CAD build for the part. Positions are in the model's coordinates, mm. Coordinates: 2 decimals unless noted, no trailing zeros. Write each loop counter-clockwise with the first axis right and the second up, starting at its lowest first coordinate (ties: lowest second). Pieces come first, ordered by that corner, then holes. Notation, with made-up numbers: (-13, -16.75) - (18, -16.75) arc R27 cw to (18, 6.25) - close; hole circle Ø5 at (29.25, 57). An arc over 180 degrees is marked (long way). Answer in a Markdown table with one row per item. Add a question column.
Q1. Pin check, flat tip, straight feed: pin 1 (1 mm diameter, centred on y = -1, z = 10.5, fed in from +X). Stop position of the tip, or through.
Q2. Band-saw the part on A-A (z = 18.75). List the corners of the cut face in (x, y).
Q3. Band-saw the part on C-C (y = 0.45). List the corners of the cut face in (x, z), and give its area (3 significant figures).
Q4. Band-saw the part on B-B (x = 0.3). List the corners of the cut face in (y, z), and give its area (3 significant figures).
Q5. Drill centre lines: line 1 along Y through (x, z) = (0.05, 20.5); line 2 along Y through (x, z) = (-0.7, 16). Where is each one in solid material? Low to high. Write a range as from..to.
Autodesk Fusion 360 part; units mm, degrees
sketch "Boceto1" plane through (0, 0, 0) normal (0, 0, 1) x (1, 0, 0)
  line L0 (0, 0) -> (120, 0)
  line L1 (120, 0) -> (120, 50)
  line L2 (120, 50) -> (0, 50)
  line L3 (0, 50) -> (0, 0)
  dimension "d1" = 120
  dimension "d2" = 50
extrude "Extruir1" add sketch "Boceto1" along normal blind 3
sketch "Boceto2" plane through (0, 0, 3) normal (0, 0, 1) x (-1, 0, 0)
  line L0 (0, -50) -> (0, 0)
  line L1 (0, 0) -> (-120, 0)
  line L2 (-120, 0) -> (-120, -50)
  line L3 (-120, -50) -> (0, -50)
  line L4 (-120, -25) -> (0, -25)
  line L5 (-120, -25) -> (-100, -25)
  circle A0 centre (-100, -25) radius 3
  line L6 (-100, -25) -> (-83.13, -25)
  circle A1 centre (-83.13, -25) radius 3
  line L7 (-83.13, -25) -> (-66.26, -25)
  circle A2 centre (-66.26, -25) radius 3
  line L8 (-66.26, -25) -> (-49.39, -25)
  circle A3 centre (-49.39, -25) radius 3
  line L9 (-49.39, -25) -> (-32.52, -25)
  circle A4 centre (-32.52, -25) radius 3
  line L10 (-32.52, -25) -> (-15.65, -25)
  circle A5 centre (-15.65, -25) radius 3
  dimension "d5" = 20
  dimension "d6" = 6
  dimension "d7" = 16.87
  dimension "d8" = 6
  dimension "d9" = 16.87
  dimension "d11" = 6
  dimension "d12" = 16.87
  dimension "d13" = 6
  dimension "d14" = 16.87
  dimension "d15" = 6
  dimension "d16" = 16.87
  dimension "d17" = 6
extrude "Extruir2" cut sketch "Boceto2" against normal blind 3 contours L4 L10 A5 | L4 L10 A5 | L4 L5 A0 L6 | L4 L5 A0 L6 | L4 L9 A4 L10 | L4 L9 A4 L10 | L4 L6 A1 L7 | L4 L6 A1 L7 | L4 L8 A3 L9 | L4 L8 A3 L9 | L4 L7 A2 L8 | L4 L7 A2 L8
equation "d6 = D_b"
equation "d7 = Dc"
equation "d8 = D_b"
equation "d9 = Dc"
equation "Dc = 16.87 mm"
equation "d11 = D_b"
equation "d12 = Dc"
equation "d13 = D_b"
equation "d14 = Dc"
equation "d15 = D_b"
equation "d16 = Dc"
equation "d17 = D_b"
equation "D_b = 6 mm"

Autodesk Fusion 360 part; units mm, degrees
sketch "Boceto1" plane through (0, 0, 0) normal (0, 0, 1) x (1, 0, 0)
  circle A0 centre (0, 0) radius 1
  dimension "d1" = 2
extrude "Extruir1" add sketch "Boceto1" along normal blind 25
Checked values:
| question | item | result |
|---|---|---|
| 1 | pin 1 | stops at x = 0.87 |
| 2 | outline | circle Ø2 at (0, 0) |
| 3 | outline | (-0.89, 0) - (0.89, 0) - (0.89, 25) - (-0.89, 25) - close |
| 3 | area | 44.7 mm² |
| 4 | outline | (-0.95, 0) - (0.95, 0) - (0.95, 25) - (-0.95, 25) - close |
| 4 | area | 47.7 mm² |
| 5 | line 1 | y = -1..1 |
| 5 | line 2 | y = -0.71..0.71 |
